Part model, mm, in its own coordinate system. Coordinates: 2 decimals unless noted, no trailing zeros. Loops run counter-clockwise (first coordinate to the right, second up) from the corner with the lowest first, then second, coordinate; pieces in that order, holes last. Notation, with made-up numbers: M 40,-37.5 L 50,-37.5 A32 ccw 50,-6.5 Z; hole C 18,18 d6. An arc over 180 degrees is marked long. Use a Markdown table: item, result. Add a question column.
1) Pin check, flat tips, straight feed: pin 1 Ø1.5 at (x, y) = (38.5, -1) entering from -Z; pin 2 Ø0.9 at (x, y) = (13, -2) entering from -Z; pin 3 Ø2.5 at (x, z) = (0, 0) entering from +Y. Stop position of each tip, or through.
2) Band-saw the part on A-A (y = -0.55). List the corners of the cut face in (x, z), plus the area to 3 significant figures.
3) Wall check: probe 1 along X at (y, z) = (-2.4, 53); probe 2 along Z at (x, y) = (46, -0.35); probe 3 along Z at (x, y) = (10, -1.1). Give the ranges that are in metal, low to high. Write a range as from..to.
4) Band-saw the part on B-B (x = 29). List the corners of the cut face in (y, z), plus the area to 3 significant figures.
5) Band-saw the part on C-C (z = 27.5). List the corners of the cut face in (x, y), plus the area to 3 significant figures.
from build123d import *

# Parameters (mm, degrees)
F0_R     = 2.1
F1_DEPTH = 3


with BuildPart() as f1:
    # F0 (on Front) → F1 (new body)
    with BuildSketch(Plane.XZ):
        with BuildLine():
            Line((70, -72.5), (250, -72.5))
            ThreePointArc((250, -72.5), (260.606602, -68.106602), (265, -57.5))
            Line((265, -57.5), (265, 57.5))
            ThreePointArc((265, 57.5), (260.606602, 68.106602), (250, 72.5))
            Line((250, 72.5), (70, 72.5))
            ThreePointArc((70, 72.5), (59.393398, 68.106602), (55, 57.5))
            Line((55, 57.5), (55, 15.4))
            Line((55, 15.4), (55, 12.4))
            Line((55, 12.4), (20, 12.4))
            Line((20, 12.4), (20, 9.4))
            Line((20, 9.4), (0, 9.4))
            ThreePointArc((0, 9.4), (-3.535534, 7.935534), (-5, 4.4))
            Line((-5, 4.4), (-5, 0))
            Line((-5, 0), (-5, -4.4))
            ThreePointArc((-5, -4.4), (-3.535534, -7.935534), (0, -9.4))
            Line((0, -9.4), (20, -9.4))
            Line((20, -9.4), (20, -12.4))
            Line((20, -12.4), (55, -12.4))
            Line((55, -12.4), (55, -57.5))
            ThreePointArc((55, -57.5), (59.393398, -68.106602), (70, -72.5))
        make_face()
        Circle(F0_R, mode=Mode.SUBTRACT)
    extrude(amount=F1_DEPTH)


solid = f1.part
Entries:
| question | item | result |
|---|---|---|
| 1 | pin 1 | z = -12.4 |
| 1 | pin 2 | z = -9.4 |
| 1 | pin 3 | through |
| 2 | outline | M -5,-4.4 A5 ccw 0,-9.4 L 20,-9.4 L 20,-12.4 L 55,-12.4 L 55,-57.5 A15 ccw 70,-72.5 L 250,-72.5 A15 ccw 265,-57.5 L 265,57.5 A15 ccw 250,72.5 L 70,72.5 A15 ccw 55,57.5 L 55,12.4 L 20,12.4 L 20,9.4 L 0,9.4 A5 ccw -5,4.4 Z; hole C 0,0 d4.2 |
| 2 | area | 31,600 mm2 |
| 3 | probe 1 | 55..265 |
| 3 | probe 2 | -12.4..12.4 |
| 3 | probe 3 | -9.4..9.4 |
| 4 | outline | M -3,-12.4 L 0,-12.4 L 0,12.4 L -3,12.4 Z |
| 4 | area | 74.4 mm2 |
| 5 | outline | M 55,-3 L 265,-3 L 265,0 L 55,0 Z |
| 5 | area | 630 mm2 |
